```python
from build123d import *

# Parameters (mm, degrees)
F0_R            = 15
F0_R_2          = 11
F0_R_3          = 7.5
F1_DEPTH        = 4
F2_DEPTH        = 20
F4_ANGLE_BACK   = 5
F4_ANGLE        = 10
F4_COPIES_COUNT = 8
F5_SIZE         = 1


# Not quite as in the source:
# - a pattern or mirror of a feature is missing from the dataset's text; its kind, count and spacing are read off the source's solid


with BuildPart() as f1:
    # F0 (on Top) → F1 (new body)
    with BuildSketch(Plane.XY):
        Circle(F0_R)
        Circle(F0_R_2, mode=Mode.SUBTRACT)
        Circle(F0_R_2)
        Circle(F0_R_3, mode=Mode.SUBTRACT)
        Circle(F0_R_3)
    extrude(amount=-F1_DEPTH)

    # F0 (on Top) → F2 (join)
    with BuildSketch(Plane.XY):
        Circle(F0_R)
        Circle(F0_R_2, mode=Mode.SUBTRACT)
        Circle(F0_R_3)
    extrude(amount=F2_DEPTH)

    # F3 (on Front) → F4 (revolve)
    with BuildSketch(Plane.XZ, mode=Mode.PRIVATE) as f4_sk:
        Polygon((0, 20), (0, 0), (7.5, 0), (10.3, 8), (7.5, 20), align=None)
    f4 = revolve(f4_sk.sketch.rotate(Axis((0, 0, 10), (0, 0, 1)), -F4_ANGLE_BACK), axis=Axis((0, 0, 10), (0, 0, 1)), revolution_arc=F4_ANGLE)

    # F4_copies: F4 ×8 about axis
    f4_copies_axis = Axis((0, 0, 0), (0, 0, 1))
    for i in range(1, F4_COPIES_COUNT):
        add(f4.rotate(f4_copies_axis, i * 360 / F4_COPIES_COUNT))

    # F5
    f5_edges = [f1.edges().sort_by_distance(p)[0] for p in [
        (-15, 0, 20),
        (-11, 0, 20),
        (-15, 0, -4),
    ]]
    chamfer(f5_edges, length=F5_SIZE)


solid = f1.part
```
The listing builds one solid part. Answer for the finished solid, in the listing's coordinates (mm). A direction names the side the tool comes from. Coordinates: 2 decimals unless noted, no trailing zeros. Write each loop counter-clockwise with the first axis right and the second up, starting at its lowest first coordinate (ties: lowest second). Pieces come first, ordered by that corner, then holes. Notation, with made-up numbers: (-34.5, 31) - (-29.5, 31) arc R23 ccw to (-29.5, 52) - close; hole circle Ø9 at (21.25, 37). An arc over 180 degrees is marked (long way). Return JSON: item names as keys, results as strings. Group by question number.
Q1. The part is cut by section B-B on x = 0. Write down the section's boundary in (y, z), and give its area (3 significant figures).
Q2. Which of the six approach directions +Z, -Z, +X, -X, +Y, -Y give full straight-line access (tool end or side, diameter ignored) to faces 1 (the flat face through (7.2, 2.6, 0)), 2 (the cylindrical face through (6.917, -2.9, 9.86))?
Q3. The part is cut by section A-A on z = 3. State how many separate pieces and enclosed holes the cut face has, and give its area (3 significant figures).
Q4. Find the intervals of material crossed by line 1 along Y through (x, z) = (6.5, 8.5); line 2 along Y through (x, z) = (0, 10); line 3 along X through (y, z) = (-8.25, 10), in increasing order. Write a range as [from, to].
Q5. Flat-ended cylindrical pins translate along their axes: pin 1 Ø12 at (y, z) = (-3, 10) entering from -X; pin 2 Ø1.5 at (x, z) = (-8, 5.5) entering from -Y; pin 3 Ø3 at (x, z) = (8, 0) entering from -Y; pin 4 Ø5 at (y, z) = (9, 5.5) entering from -X. Find the tip coordinate at first contact, or state that the pin passes through.
Evaluation:
{
 "1": {"outline": "(-15, -3) - (-14, -4) - (14, -4) - (15, -3) - (15, 19) - (14, 20) - (12, 20) - (11, 19) - (11, 0) - (7.5, 0) - (10.3, 8) - (7.5, 20) - (-7.5, 20) - (-10.3, 8) - (-7.5, 0) - (-11, 0) - (-11, 19) - (-12, 20) - (-14, 20) - (-15, 19) - close", "area": "633 mm2"},
 "2": {"face 1": "none", "face 2": "+Z"},
 "3": {"separate pieces": "2", "enclosed holes": "1", "area": "515 mm2"},
 "4": {"line 1": "y = [-13.52, -8.87], [-7.75, -5.45], [-3.74, 3.74], [5.45, 7.75], [8.87, 13.52]", "line 2": "y = [-15, -11], [-9.83, 9.83], [11, 15]", "line 3": "x = [-12.53, -7.28], [-0.72, 0.72], [7.28, 12.53]"},
 "5": {"pin 1": "stops at x = -15", "pin 2": "stops at y = -13.13", "pin 3": "stops at y = -13.52", "pin 4": "stops at x = -13.52"}
}
